Source: CAD feature listing. Evaluate the final solid. Frame: model axes, mm. Face numbers are marked on the shaded views. A direction names the side the tool comes from. Coordinates: 2 decimals unless noted, no trailing zeros. Order: outer loops, then holes, each group sorted by start corner. A loop starts at its lowest first (then second) coordinate and runs counter-clockwise, first axis right, second up.
```python
from build123d import *

# Parameters (mm, degrees)
BOSS_EXTRUDE1_DEPTH = 1
BOSS_EXTRUDE2_START = -5
SKETCH2_R           = 4
BOSS_EXTRUDE2_DEPTH = 20
BOSS_EXTRUDE3_DEPTH = 20
CIRPATTERN1_COUNT   = 6
CIRPATTERN1_ANGLE   = 150
CIRPATTERN2_COUNT   = 7
CIRPATTERN2_ANGLE   = 180


with BuildPart() as part:
    # Sketch1 → Boss-Extrude1 (new body)
    with BuildSketch(Plane.XY):
        Polygon((0, 0), (0, 20), (2, 20), (2, 395), (32.628445402, 395), (82, 115), (82, -5), (2, -5), (2, 0), align=None)
    boss_extrude1 = extrude(amount=BOSS_EXTRUDE1_DEPTH)



with BuildPart() as body_2:
    # Sketch2 → Boss-Extrude2 (new body)
    with BuildSketch(Plane.XZ.offset(5).offset(BOSS_EXTRUDE2_START)):
        with Locations((-5, 0.5)):
            Circle(SKETCH2_R)
    extrude(amount=-BOSS_EXTRUDE2_DEPTH)


with BuildPart() as part_1:
    add(part.part)

    add(body_2.part)  # Boss-Extrude3 merges body 2
    # Sketch3 → Boss-Extrude3 (add)
    with BuildSketch(Plane.XZ):
        with BuildLine():
            Line((0, 1), (-1.136296695, 1.53527618))
            ThreePointArc((-1.136296695, 1.53527618), (-1, 0.5), (-1.136296695, -0.53527618))
            Line((-1.136296695, -0.53527618), (0, 0))
            Line((0, 0), (0, 1))
        make_face()
    boss_extrude3 = extrude(amount=-BOSS_EXTRUDE3_DEPTH)

    # CirPattern1: Boss-Extrude3 ×6 about axis
    cirpattern1_axis = Axis((-5, 0, 0.5), (0, 1, 0))
    for i in range(1, CIRPATTERN1_COUNT):
        add(boss_extrude3.rotate(cirpattern1_axis, i * CIRPATTERN1_ANGLE / (CIRPATTERN1_COUNT - 1)))

    # CirPattern2: Boss-Extrude1 ×7 about axis, 1 skipped
    cirpattern2_axis = Axis((-5, 0, 0.5), (0, 1, 0))
    add([boss_extrude1.rotate(cirpattern2_axis, i * CIRPATTERN2_ANGLE / (CIRPATTERN2_COUNT - 1)) for i in range(1, CIRPATTERN2_COUNT) if i not in (6,)])


solid = part_1.part
```
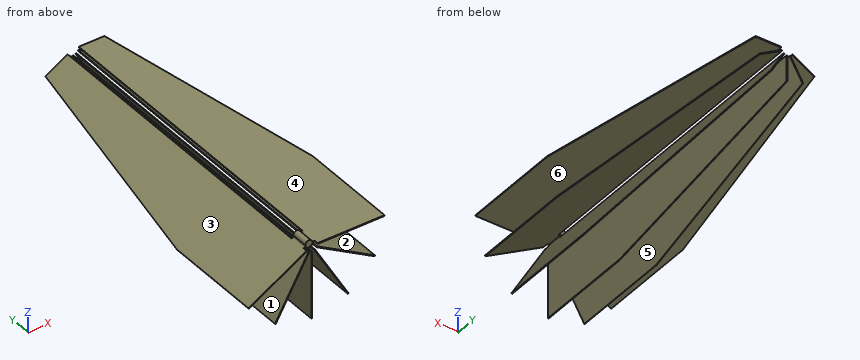
1. Material intervals for line 1 along Z through (x, y) = (28, 138.5); line 2 along X through (y, z) = (216.5, -8.5); line 3 along Z through (x, y) = (10.5, 83), sorted ascending.
2. Section query D-D, the plane y = 167. Output: boundary loops of the cut face in (x, z), plus the area to 3 significant figures.
3. Section query B-B, the plane x = -18. Output: boundary loops of the cut face in (y, z).
4. Contact query for flat-ended pins moving along their axis: P1, Ø8, axis at x = 59.5, y = 257.5, coming from the -Z side; P2, Ø3, axis at y = 254, z = -10.5, coming from the +X side; P3, Ø0.5, axis at y = 120, z = 0.5, coming from the -X side. Output: stop coordinate, or through.
5. Access query for the marked faces 1, 2 and 3. Directions: +Z, -Z, +X, -X, +Y, -Y. A direction counts if a zero-diameter tool reaches every point of the face in a straight line with its end or side. Return the directions, or none.
6. Draft query along Z for the marked faces 4, 5 and 6. Return one class per face: +Z half, -Z half, draft (parallel to the pull), parting line (faces both ways), or undercut.
7. Section query A-A, the plane y = 53. Output: boundary loops of the cut face in (x, z), plus the area to 3 significant figures.
8. Section query C-C, the plane z = -50. Output: boundary loops of the cut face in (x, y).
Answer key:
1. line 1: z = -57.66 to -55.66, -19.13 to -17.98, 0 to 1
1. line 2: x = -21.59 to -19.59, -10.77 to -9.62, -5.5 to -4.5, -0.38 to 0.77, 9.59 to 11.59
1. line 3: z = -27.35 to -25.35, -9.03 to -7.87, 0 to 1
2. outline: (-72.65, -37.98) - (-72.15, -38.85) - (-10.81, -3.43) - (-11.31, -2.57) - close; (-44.35, -66.65) - (-43.48, -67.15) - (-8.07, -5.81) - (-8.93, -5.31) - close; (-5.5, -77.33) - (-4.5, -77.33) - (-4.5, -6.5) - (-5.5, -6.5) - close; (-1.93, -5.81) - (33.48, -67.15) - (34.35, -66.65) - (-1.07, -5.31) - close; (0.81, -3.43) - (62.15, -38.85) - (62.65, -37.98) - (1.31, -2.57) - close; (2, 0) - (72.83, 0) - (72.83, 1) - (2, 1) - close
2. area: 425 mm2
3. outline: (-5, -23.02) - (395, -23.02) - (395, -21.02) - (-5, -21.02) - close; (-5, -7.58) - (395, -7.58) - (395, -6.43) - (-5, -6.43) - close
4. P1: stops at z = 0
4. P2: stops at x = 17.65
4. P3: stops at x = 2
5. face 1: +Y, -Y
5. face 2: +X, +Y, -Y
5. face 3: +Z, -X, +Y, -Y
6. face 4: +Z half
6. face 5: -Z half
6. face 6: undercut
7. outline: (-80.59, -42.57) - (-80.09, -43.43) - (-10.81, -3.43) - (-11.31, -2.57) - close; (-48.93, -74.59) - (-48.07, -75.09) - (-8.07, -5.81) - (-8.93, -5.31) - close; (-5.5, -86.5) - (-4.5, -86.5) - (-4.5, -6.5) - (-5.5, -6.5) - close; (-1.93, -5.81) - (38.07, -75.09) - (38.93, -74.59) - (-1.07, -5.31) - close; (0.81, -3.43) - (70.09, -43.43) - (70.59, -42.57) - (1.31, -2.57) - close; (2, 0) - (82, 0) - (82, 1) - (2, 1) - close
7. area: 480 mm2
8. outline: (-34.73, -5) - (-33.58, -5) - (-33.58, 279.33) - (-34.73, 276.06) - close; (-5.5, -5) - (-4.5, -5) - (-4.5, 322) - (-5.5, 322) - close; (23.58, -5) - (24.73, -5) - (24.73, 276.06) - (23.58, 279.33) - close
